Here's how the part is built. I have some questions about the finished solid (model axes, mm). Give positions to 0.01 mm unless a question says otherwise; leave off trailing zeros. Loops run counter-clockwise (first coordinate to the right, second up) from the corner with the lowest first, then second, coordinate; pieces in that order, holes last.
Q1. If we section it at A-A (y = 2.5): Please give me the cut outline in (x, z), plus the area to 3 significant figures.
Q2. I need wall thicknesses on line 1 (X direction, y = 2.5, z = -5.5); line 2 (X direction, y = 6, z = -5); line 3 (Y direction, x = -160, z = -5.5). Which ranges of each line are inside material? Lowest first, please.
Q3. If we section it at C-C (z = -2.75): Please give me the cut outline in (x, y).
Q4. If we section it at D-D (x = -57): Please give me the cut outline in (y, z).
Q5. If we section it at B-B (x = 160): Please give me the cut outline in (y, z), plus the area to 3 significant figures.
Q6. We'd pull the mould along X, two halves only. Please class faces 1 (the face through (-3, 17.5, -4)), 2 (the face through (-196.99, 14.65, -3.94)), 3 (the face through (163.815, 3.701, -3.944)), 4 (the face through (200, -5, -4)): +X half, -X half, draft (parallel to the pull), parting line (faces both ways), or undercut.
Autodesk Inventor part; units mm, degrees
ref_plane "YZ Plane" through (0, 0, 0) normal (1, 0, 0) x (0, 1, 0)
ref_plane "XZ Plane" through (0, 0, 0) normal (0, 1, 0) x (-1, 0, 0)
ref_plane "XY Plane" through (0, 0, 0) normal (0, 0, 1) x (1, 0, 0)
sketch "Sketch1" plane through (0, 0, 0) normal (0, 0, 1) x (1, 0, 0)
  line L0 (0, 26.9853) -> (0, -24.9142)
  line L1 (-282.8995, 0) -> (282.8995, 0)
  line L2 (-190, 17.5) -> (190, 17.5)
  line L3 (200, 7.5) -> (200, -17.5)
  line L4 (200, -17.5) -> (-200, -17.5)
  line L5 (-200, -17.5) -> (-200, 7.5)
  arc A0 (-190, 17.5) -> (-200, 7.5) centre (-190, 7.5) ccw
  arc A1 (200, 7.5) -> (190, 17.5) centre (190, 7.5) ccw
  circle A2 centre (-160, 2.5) radius 4
  circle A3 centre (160, 2.5) radius 4
  point P0 (0, 0)
  point P1 (-200, 17.5)
  point P2 (200, 17.5)
  dimension "d0" = 35
  dimension "d1" = 400
  dimension "d2" = 10
  dimension "d3" = 8
  dimension "d4" = 160
  dimension "d5" = 20
extrude "Extrusion1" add sketch "Sketch1" against normal blind 8 contours L2 A1 L3 L1 A3 L0 | L0 L1 A2 L5 A0 L2 | L1 A3 L3 L4 L0 | L0 L4 L5 L1 A2
chamfer "Chamfer1" distance 4 angle 45 1 edges at (0, -17.5, 0)
properties part number "SlipersLåda 211018009"
Check sheet entries:
1. outline: (-200, -8) - (-164, -8) - (-164, 0) - (-200, 0) - close; (-156, -8) - (156, -8) - (156, 0) - (-156, 0) - close; (164, -8) - (200, -8) - (200, 0) - (164, 0) - close
1. area: 3,070 mm2
2. line 1: x = -200 to -164, -156 to 156, 164 to 200
2. line 2: x = -200 to -161.94, -158.06 to 158.06, 161.94 to 200
2. line 3: y = -17.5 to -1.5, 6.5 to 17.5
3. outline: (-200, -16.25) - (200, -16.25) - (200, 7.5) arc R10 ccw to (190, 17.5) - (-190, 17.5) arc R10 ccw to (-200, 7.5) - close; hole circle Ø8 at (-160, 2.5); hole circle Ø8 at (160, 2.5)
4. outline: (-17.5, -8) - (17.5, -8) - (17.5, 0) - (-13.5, 0) - (-17.5, -4) - close
5. outline: (-17.5, -8) - (-1.5, -8) - (-1.5, 0) - (-13.5, 0) - (-17.5, -4) - close; (6.5, -8) - (17.5, -8) - (17.5, 0) - (6.5, 0) - close
5. area: 208 mm2
6. face 1: draft
6. face 2: -X half
6. face 3: undercut
6. face 4: +X half
